Autodesk Inventor part; units mm, degrees
ref_plane "YZ Plane" through (0, 0, 0) normal (1, 0, 0) x (0, 1, 0)
ref_plane "XZ Plane" through (0, 0, 0) normal (0, 1, 0) x (-1, 0, 0)
ref_plane "XY Plane" through (0, 0, 0) normal (0, 0, 1) x (1, 0, 0)
sketch "Sketch1" plane through (0, 0, 0) normal (0, 0, 1) x (1, 0, 0)
  line L0 (0, 0) -> (0, 15.875)
  line L1 (0, 15.875) -> (0.7937, 15.875)
  line L2 (0.7937, 15.875) -> (0.7938, 0.7937)
  line L3 (0.7938, 0.7937) -> (15.875, 0.7937)
  line L4 (15.875, 0.7937) -> (15.875, 0)
  line L5 (15.875, 0) -> (0, 0)
  dimension "d0" = 15.875
  dimension "d1" = 0.7937
extrude "Extrusion1" add sketch "Sketch1" along normal blind 127
sketch "Sketch2" plane through (0, 0, 0) normal (0, -1, 0) x (1, 0, 0)
  line L0 (15.875, 0) -> (0, 0)
  line L1 (0, 127) -> (15.875, 127)
  line L2 (7.9375, 127) -> (7.9375, 0) construction
  circle A0 centre (7.9375, 117.475) radius 1.5875
  circle A1 centre (7.9375, 9.525) radius 1.5875
  dimension "d4" = 3.175
  dimension "d5" = 3.175
  dimension "d6" = 9.525
  dimension "d7" = 9.525
extrude "Extrusion2" cut sketch "Sketch2" against normal through all
sketch "Sketch3" plane through (0, 0, 0) normal (-1, 0, 0) x (0, 0, 1)
  line L0 (0, 0) -> (0, 15.875)
  line L1 (127, 15.875) -> (127, 0)
  line L2 (0, 7.9375) -> (127, 7.9375) construction
  circle A0 centre (9.525, 7.9375) radius 1.5875
  circle A1 centre (117.475, 7.9375) radius 1.5875
  dimension "d10" = 3.175
  dimension "d11" = 3.175
  dimension "d12" = 9.525
  dimension "d13" = 9.525
extrude "Extrusion3" cut sketch "Sketch3" against normal through all
properties part number "Shooter Wheel Shields Connector Bar" material "Aluminum 6061"
CAD build for the part. Positions are in the model's coordinates, mm. A direction names the side the tool comes from. Give positions to 0.01 mm unless a question says otherwise; leave off trailing zeros. Loops run counter-clockwise (first coordinate to the right, second up) from the corner with the lowest first, then second, coordinate; pieces in that order, holes last. Notation, with made-up numbers: M 39,71.25 L 51,71.25 A14 ccw 51,96.25 Z; hole C 56,15 d3. An arc over 180 degrees is marked long. Use one line per item in the form item = value.
Item 1: Flat gauge pins, fed straight in: pin 1 (4 mm diameter, centred on y = 7.94, z = 117.48, fed in from +X); pin 2 (3.5 mm diameter, centred on x = 7.94, z = 9.52, fed in from +Y). Where does each tip first touch, or does it go through?
Determined:
pin_1 = 0.79
pin_2 = 0.79
Item 2: Slice it at C-C (y = 14.75). List the corners of the cut face in (x, z), plus the area to 3 significant figures.
Determined:
outline = M 0,0 L 0.79,0 L 0.79,127 L 0,127 Z
area = 101 mm2
Item 3: Drill centre line: probe 1 along Y at (x, z) = (8, 46). Where is it in solid material? Low to high. Write a range as from..to.
Determined:
probe_1 = 0..0.79
Item 4: Slice it at A-A (z = 77.5). List the corners of the cut face in (x, y) (3 decimals).
Determined:
outline = M 0,0 L 15.875,0 L 15.875,0.794 L 0.794,0.794 L 0.794,15.875 L 0,15.875 Z
Item 5: Slice it at B-B (x = 7.75). List the corners of the cut face in (y, z).
Determined:
outline = M 0,0 L 0.79,0 L 0.79,7.95 L 0,7.95 Z; M 0,11.1 L 0.79,11.1 L 0.79,115.9 L 0,115.9 Z; M 0,119.05 L 0.79,119.05 L 0.79,127 L 0,127 Z
Item 6: Which spindle directions (+Z, -Z, +X, -X, +Y, -Y) get a long thin tool onto all of the face, cutting with end or side? Do faces 1 (the face through (7.73, 0.39, 119.05)), 2 (the face through (8, 0.794, 63)). Say none if no direction does.
Determined:
face_1 = +Y, -Y
face_2 = +Z, -Z, +X, +Y
Item 7: Two-plate mould, pull along Z, no slides. Class faces 3 (the face through (4.4, 0.3, 0)), 4 (the face through (8.67, 0.391, 8.117)), 5 (the face through (0, 8, 63)): pulls with the +Z half, pulls with the -Z half, needs draft (parallel to the pull), parting line crosses it, or undercut.
Determined:
face_3 = pulls with the -Z half
face_4 = undercut
face_5 = needs draft
